```python
from build123d import *

# Parameters (mm, degrees)
SKETCH1_W               = 3.05
SKETCH1_H               = 20
SKETCH1_W_2             = 15.818181818
SKETCH1_H_2             = 3
BOSS_EXTRUDE1_DEPTH     = 3
CUT_EXTRUDE9_DEPTH      = 1
CUT_EXTRUDE9_DEPTH_BACK = 4
FILLET3_R               = 2.5
CUT_EXTRUDE8_DEPTH      = 4
CUT_EXTRUDE8_DEPTH_BACK = 1


with BuildPart() as part:
    # Sketch1 → Boss-Extrude1 (new body)
    with BuildSketch(Plane.XY):
        Polygon((-90, 50), (-90, -50), (-71.181818182, -50), (-55.363636364, -50), (-39.545454545, -50), (-23.727272727, -50), (-7.909090909, -50), (7.909090909, -50), (23.727272727, -50), (39.545454545, -50), (55.363636364, -50), (71.181818182, -50), (90, -50), (90, 50), align=None)
        with Locations((-85.475, -20)):
            Rectangle(SKETCH1_W, SKETCH1_H, mode=Mode.SUBTRACT)
        with Locations((85.475, -20)):
            Rectangle(SKETCH1_W, SKETCH1_H, mode=Mode.SUBTRACT)
        with Locations((-85.475, 20)):
            Rectangle(SKETCH1_W, SKETCH1_H, mode=Mode.SUBTRACT)
        with Locations((85.475, 20)):
            Rectangle(SKETCH1_W, SKETCH1_H, mode=Mode.SUBTRACT)
        with Locations((-63.272727273, -51.5)):
            Rectangle(SKETCH1_W_2, SKETCH1_H_2)
        with Locations((-31.636363636, -51.5)):
            Rectangle(SKETCH1_W_2, SKETCH1_H_2)
        with Locations((0, -51.5)):
            Rectangle(SKETCH1_W_2, SKETCH1_H_2)
        with Locations((31.636363636, -51.5)):
            Rectangle(SKETCH1_W_2, SKETCH1_H_2)
        with Locations((63.272727273, -51.5)):
            Rectangle(SKETCH1_W_2, SKETCH1_H_2)
    extrude(amount=BOSS_EXTRUDE1_DEPTH)

    # Sketch7 → Cut-Extrude9 (cut, two sides)
    with BuildSketch(Plane.XY.offset(3)) as cut_extrude9_sk:
        Polygon((-78.252607778, 50), (-42.5, 20), (42.5, 20), (78.252607778, 50), align=None)
    extrude(amount=CUT_EXTRUDE9_DEPTH, mode=Mode.SUBTRACT)
    extrude(cut_extrude9_sk.sketch, amount=-CUT_EXTRUDE9_DEPTH_BACK, mode=Mode.SUBTRACT)

    # Fillet3
    fillet3_edges = [part.edges().sort_by_distance(p)[0] for p in [
        (-78.252607778, 50, 1.5),
        (78.252607778, 50, 1.5),
        (42.5, 20, 1.5),
        (-42.5, 20, 1.5),
        (-90, 50, 1.5),
        (90, 50, 1.5),
    ]]
    fillet(fillet3_edges, radius=FILLET3_R)

    # Sketch6 → Cut-Extrude8 (cut, two sides)
    with BuildSketch(Plane.XY) as cut_extrude8_sk:
        Polygon((-67.83865663, 10.5), (-78, 10.5), (-78, -24.5), (-67.83865663, -24.5), (-57.735026919, -7), align=None)
        Polygon((-59.178402592, -29.5), (-54.270925304, -38), (-23.671361037, -38), (-18.763883749, -29.5), (-28.867513459, -12), (-49.074772881, -12), align=None)
        Polygon((-67.83865663, -34.5), (-78, -34.5), (-78, -38), (-65.817930688, -38), align=None)
        Polygon((-10.103629711, -34.5), (-12.124355653, -38), (12.124355653, -38), (10.103629711, -34.5), align=None)
        Polygon((18.763883749, -29.5), (23.671361037, -38), (54.270925304, -38), (59.178402592, -29.5), (49.074772881, -12), (28.867513459, -12), align=None)
        Polygon((78, -38), (78, -34.5), (67.83865663, -34.5), (65.817930688, -38), align=None)
        Polygon((78, -24.5), (78, 10.5), (67.83865663, 10.5), (57.735026919, -7), (67.83865663, -24.5), align=None)
        Polygon((11.547005384, 8), (-11.547005384, 8), (-20.207259422, -7), (-10.103629711, -24.5), (10.103629711, -24.5), (20.207259422, -7), align=None)
        Polygon((-46.867642811, 8), (-58.077745879, 17.406393349), (-59.178402592, 15.5), (-49.074772881, -2), (-28.867513459, -2), (-23.094010768, 8), align=None)
        Polygon((46.867642811, 8), (23.094010768, 8), (28.867513459, -2), (49.074772881, -2), (59.178402592, 15.5), (58.077745879, 17.406393349), align=None)
        Polygon((-67.83865663, 20.5), (-65.856365013, 23.933429796), (-65.935700293, 24), (-78, 24), (-78, 20.5), align=None)
        Polygon((65.935700293, 24), (65.856365013, 23.933429796), (67.83865663, 20.5), (78, 20.5), (78, 24), align=None)
    extrude(amount=CUT_EXTRUDE8_DEPTH, mode=Mode.SUBTRACT)
    extrude(cut_extrude8_sk.sketch, amount=-CUT_EXTRUDE8_DEPTH_BACK, mode=Mode.SUBTRACT)


solid = part.part
```
The listing builds one solid part. Answer for the finished solid, in the listing's coordinates (mm). A direction names the side the tool comes from. Give positions to 0.01 mm unless a question says otherwise; leave off trailing zeros. Order: outer loops, then holes, each group sorted by start corner. A loop starts at its lowest first (then second) coordinate and runs counter-clockwise, first axis right, second up. Notation, with made-up numbers: (44, 46) - (61, 46) arc R10 cw to (61, 56) - close; hole circle Ø2 at (60, 70). An arc over 180 degrees is marked (long way). Answer in a Markdown table with one row per item. Add a question column.
Q1. The part is cut by section C-C (z = 1.8). Give the number of separate pieces and of enclosed holes in the cut face, then the cut area to 3 significant figures.
Q2. Which of the six approach directions +Z, -Z, +X, -X, +Y, -Y give full straight-line access (tool end or side, diameter ignored) to faces 3 (the flat face through (-60.617, 35.202, 1.521)), 4 (the flat face through (-1, 11, 3)), 5 (the flat face through (-56.76, -33.69, 1.48))?
Q3. The part is cut by section A-A (x = 33.5). Determine the outline of the cut face in (y, z).
Q4. Find the intervals of material crossed by line 1 along Y through (x, z) = (38, 1); line 2 along Y through (x, z) = (-43.5, 2.5); line 3 along X through (y, z) = (-29, 1.6), in increasing order. Write a range as [from, to].
Q5. Given P1, Ø1.5, axis at x = -71.5, z = 1.5, coming from the +Y side; P2, Ø1.5, axis at y = -51.5, z = 2, coming from the +X side; P3, Ø0.9, axis at x = 15, z = 1, coming from the -Y side, each flat-ended and moving along its own axis, determine where each tip first touches the part or whether it passes through.
Q6. For a pull along X with two mould halves and no side action, classify faces 1 (the flat face through (25.94, 3.07, 1.48)), 2 (the flat face through (-1, 11, 0)) as released by +X, released by -X, zero draft, split by the parting line, or undercut.
Q7. The part is cut by section B-B (y = 37). Determine the outline of the cut face in (x, z), then the cut area to 3 significant figures.
Determined:
| question | item | result |
|---|---|---|
| 1 | separate pieces | 1 |
| 1 | enclosed holes | 16 |
| 1 | area | 9,790 mm² |
| 2 | face 3 | +Z, -Z, +Y |
| 2 | face 4 | +Z, +X, -X, +Y, -Y |
| 2 | face 5 | +Z, -Z |
| 3 | outline | (-53, 0) - (-38, 0) - (-38, 3) - (-53, 3) - close; (-12, 0) - (-2, 0) - (-2, 3) - (-12, 3) - close; (8, 0) - (20, 0) - (20, 3) - (8, 3) - close |
| 4 | line 1 | y = [-53, -38], [-12, -2], [8, 20] |
| 4 | line 2 | y = [-50, -38], [-12, -2], [8, 20.84] |
| 4 | line 3 | x = [-90, -87], [-83.95, -58.89], [-19.05, 19.05], [58.89, 83.95], [87, 90] |
| 5 | P1 | stops at y = 44.96 |
| 5 | P2 | stops at x = 71.18 |
| 5 | P3 | stops at y = -50 |
| 6 | face 1 | undercut |
| 6 | face 2 | zero draft |
| 7 | outline | (-90, 0) - (-62.76, 0) - (-62.76, 3) - (-90, 3) - close; (62.76, 0) - (90, 0) - (90, 3) - (62.76, 3) - close |
| 7 | area | 163 mm² |
